Source: three-view drawing plus pictorial views. Frame: mm from the lowest corner of the part. A direction names the side the tool comes from. Round coordinates to 2 decimals unless told otherwise and drop trailing zeros. Write each loop counter-clockwise with the first axis right and the second up, starting at its lowest first coordinate (ties: lowest second). Pieces come first, ordered by that corner, then holes. Notation, with made-up numbers: (-30.75, -24.75) -> (-9.75, -24.75) arc R19 ccw to (-9.75, 12.25) -> close; hole circle Ø4 at (-28, -4.75). An arc over 180 degrees is marked (long way). Put each result on its own line as item: value.
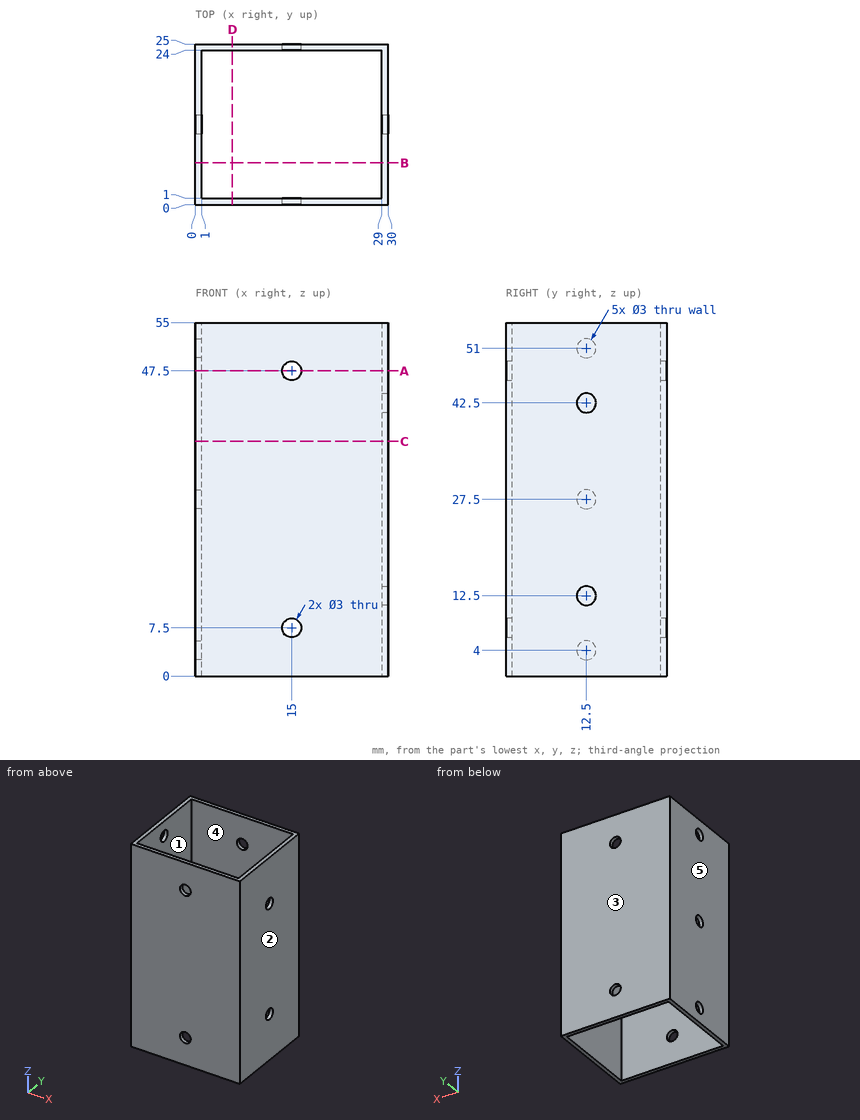
Q1. Cut plane D-D on x = 5.75. Output: boundary loops of the cut face in (y, z), and give its area (3 significant figures).
Ans:
outline: (0, 0) -> (1, 0) -> (1, 55) -> (0, 55) -> close; (24, 0) -> (25, 0) -> (25, 55) -> (24, 55) -> close
area: 110 mm^2
Q2. Cut plane A-A on z = 47.5. Output: boundary loops of the cut face in (x, y).
Ans:
outline: (0, 0) -> (13.5, 0) -> (13.5, 1) -> (1, 1) -> (1, 24) -> (13.5, 24) -> (13.5, 25) -> (0, 25) -> close; (16.5, 0) -> (30, 0) -> (30, 25) -> (16.5, 25) -> (16.5, 24) -> (29, 24) -> (29, 1) -> (16.5, 1) -> close
Q3. Draft query along X for the marked faces 1, 2 and 3. Return one class per face: +X half, -X half, draft (parallel to the pull), parting line (faces both ways), or undercut.
Ans:
face 1: undercut
face 2: +X half
face 3: draft
Q4. Pin query (flat end, axial travel): pin 1 (1.8 mm diameter, centred on x = 15, z = 7.5, fed in from -Y); pin 2 (3.5 mm diameter, centred on y = 12.5, z = 4, fed in from -X); pin 3 (1.8 mm diameter, centred on y = 12.5, z = 51, fed in from -X). Return the tip coordinate at first contact, or that it passes through.
Ans:
pin 1: passes through
pin 2: stops at x = 0
pin 3: stops at x = 29
Q5. Reachability of the marked faces 4 and 5 from +Z, -Z, +X, -X, +Y, -Y: full face, straight path, thin tool, end or side. Return the list, or none.
Ans:
face 4: +Z, -Z
face 5: +Z, -Z, -X, +Y, -Y
Q6. Cut plane C-C on z = 36.5. Output: boundary loops of the cut face in (x, y), and give its area (3 significant figures).
Ans:
outline: (0, 0) -> (30, 0) -> (30, 25) -> (0, 25) -> close; hole (1, 1) -> (29, 1) -> (29, 24) -> (1, 24) -> close
area: 106 mm^2
Q7. Cut plane B-B on y = 6.5. Output: boundary loops of the cut face in (x, z), and give its area (3 significant figures).
Ans:
outline: (0, 0) -> (1, 0) -> (1, 55) -> (0, 55) -> close; (29, 0) -> (30, 0) -> (30, 55) -> (29, 55) -> close
area: 110 mm^2
Q8. Material intervals for line 1 (X direction, y = 5.25, z = 37); line 2 (Y direction, x = 6.5, z = 47); line 3 (Y direction, x = 0.75, z = 27.5), sorted ascending. Write a range as [from, to].
Ans:
line 1: x = [0, 1], [29, 30]
line 2: y = [0, 1], [24, 25]
line 3: y = [0, 11], [14, 25]
